Input: part model. Units: mm. Frame: model coordinates. A direction names the side the tool comes from. Round coordinates to 2 decimals unless told otherwise and drop trailing zeros. Write each loop counter-clockwise with the first axis right and the second up, starting at its lowest first coordinate (ties: lowest second). Pieces come first, ordered by that corner, then holes. Notation, with made-up numbers: (-30, 66) -> (-1, 66) arc R17 cw to (-1, 80) -> close; hole circle Ø2 at (-33, -21.5). An arc over 180 degrees is marked (long way). Write item = value, one per line.
Autodesk Inventor part; units mm, degrees
ref_plane "YZ Plane" through (0, 0, 0) normal (1, 0, 0) x (0, 1, 0)
ref_plane "XZ Plane" through (0, 0, 0) normal (0, 1, 0) x (-1, 0, 0)
ref_plane "XY Plane" through (0, 0, 0) normal (0, 0, 1) x (1, 0, 0)
sketch "Sketch1" plane through (0, 0, 0) normal (0, 0, 1) x (1, 0, 0)
  circle A0 centre (29.1378, 0) radius 3.5
  arc A1 (-30.8622, 6) -> (-30.8622, -6) centre (-30.8622, 0) ccw
  arc A2 (29.1378, -6) -> (29.1378, 6) centre (29.1378, 0) ccw
  arc A3 (-30.8622, -6) -> (-27.3004, -4.8284) centre (-30.8622, 0) ccw
  line L0 (-30.8622, 0) -> (-26.6195, -4.2426) construction
  line L1 (-30.8622, 0) -> (-30.8622, -6) construction
  arc A4 (-27.3004, 4.8284) -> (-30.8622, 6) centre (-30.8622, 0) ccw
  line L2 (-30.8622, 0) -> (-26.6195, 4.2426) construction
  line L3 (-30.8622, 0) -> (-30.8622, 6) construction
  arc A5 (29.1378, 6) -> (25.576, 4.8284) centre (29.1378, 0) ccw
  line L4 (29.1378, 0) -> (24.8952, 4.2426) construction
  line L5 (29.1378, 0) -> (29.1378, 6) construction
  arc A6 (25.576, -4.8284) -> (29.1378, -6) centre (29.1378, 0) ccw
  line L6 (29.1378, 0) -> (24.8952, -4.2426) construction
  line L7 (29.1378, 0) -> (29.1378, -6) construction
  line L8 (-25.5195, 4.2426) -> (23.7951, 4.2426)
  line L9 (-25.5195, -4.2426) -> (23.7951, -4.2426)
  arc A7 (-27.3004, 4.8284) -> (-25.5195, 4.2426) centre (-25.5195, 7.2426) ccw
  arc A8 (-25.5195, -4.2426) -> (-27.3004, -4.8284) centre (-25.5195, -7.2426) ccw
  arc A9 (23.7951, 4.2426) -> (25.576, 4.8284) centre (23.7951, 7.2426) ccw
  arc A10 (25.576, -4.8284) -> (23.7951, -4.2426) centre (23.7951, -7.2426) ccw
  line L10 (33.1793, 0) -> (31.1585, -3.5)
  line L11 (31.1585, -3.5) -> (27.1171, -3.5)
  line L12 (27.1171, -3.5) -> (25.0964, 0)
  line L13 (25.0964, 0) -> (27.1171, 3.5)
  line L14 (27.1171, 3.5) -> (31.1585, 3.5)
  line L15 (31.1585, 3.5) -> (33.1793, 0)
  circle A11 centre (-30.8622, 0) radius 1
  point P0 (0, 0)
  point P1 (24.8952, 4.2426)
  dimension "d1" = 7
  dimension "d2" = 60
  dimension "d3" = 6
  dimension "d4" = 6
  dimension "d5" = 45
  dimension "d6" = 45
  dimension "d7" = 45
  dimension "d8" = 45
  dimension "d9" = 3
  dimension "d17" = 2
extrude "Extrusion2" add sketch "Sketch1" along normal blind 3
properties part number "2P.03.01.18.ZW.AileronCrank"
1) Line query: L1, parallel to X at y = 0.75, z = 1.15; L2, parallel to Y at x = -21.5, z = 2.2; L3, parallel to X at y = -2, z = 2.1. Output: solid intervals per line, ascending. Write a range as from..to.
Solutions:
L1 = -36.82..-31.52, -30.2..25.53, 32.75..35.09
L2 = -4.24..4.24
L3 = -36.52..26.25, 32.02..34.79
2) Draft query along Y for faces 6 (the face through (-1, 4.243, 1)), 7 (the face through (-1, 0, 3)), 8 (the face through (29, -3.5, 1)). Return one class per face: +Y half, -Y half, draft (parallel to the pull), parting line (faces both ways), or undercut.
Solutions:
face_6 = +Y half
face_7 = draft
face_8 = undercut
3) Cut plane B-B (y = -2.5). Return the cut outline in (x, z), and give its area (3 significant figures).
Solutions:
outline = (-36.32, 0) -> (26.54, 0) -> (26.54, 3) -> (-36.32, 3) -> close; (31.74, 0) -> (34.59, 0) -> (34.59, 3) -> (31.74, 3) -> close
area = 197 mm^2
4) Cut plane D-D (x = 8). Return the cut outline in (y, z).
Solutions:
outline = (-4.24, 0) -> (4.24, 0) -> (4.24, 3) -> (-4.24, 3) -> close
5) Access query for faces 1 (the face through (-26.444, 4.389, 1.479)), 2 (the face through (29, 3.5, 1)), 3 (the face through (-36.86, -0.13, 1.48)), 4 (the face through (-1, 0, 0)), 5 (the face through (24.72, -4.39, 1.48)). Directions: +Z, -Z, +X, -X, +Y, -Y. A direction counts if a zero-diameter tool reaches every point of the face in a straight line with its end or side. Return the directions, or none.
Solutions:
face_1 = +Z, -Z, +Y
face_2 = +Z, -Z
face_3 = +Z, -Z, -X
face_4 = -Z, +X, -X, +Y, -Y
face_5 = +Z, -Z, -Y
6) Cut plane C-C (x = 30.5). Return the cut outline in (y, z).
Solutions:
outline = (-5.84, 0) -> (-3.5, 0) -> (-3.5, 3) -> (-5.84, 3) -> close; (3.5, 0) -> (5.84, 0) -> (5.84, 3) -> (3.5, 3) -> close
7) Cut plane A-A (z = 1.55). Return the cut outline in (x, y).
Solutions:
outline = (-30.86, -6) arc R6 ccw to (-27.3, -4.83) arc R3 cw to (-25.52, -4.24) -> (23.8, -4.24) arc R3 cw to (25.58, -4.83) arc R6 ccw to (29.14, -6) arc R6 ccw to (29.14, 6) arc R6 ccw to (25.58, 4.83) arc R3 cw to (23.8, 4.24) -> (-25.52, 4.24) arc R3 cw to (-27.3, 4.83) arc R6 ccw to (-30.86, 6) arc R6 ccw to start; hole circle Ø2 at (-30.86, 0); hole (25.1, 0) -> (27.12, -3.5) -> (31.16, -3.5) -> (33.18, 0) -> (31.16, 3.5) -> (27.12, 3.5) -> close
8) First-contact query: P1, Ø1, axis at x = -28, z = 2, coming from the +Y side; P2, Ø1, axis at y = 2.5, z = 2, coming from the +X side; P3, Ø1.5, axis at x = -7.5, z = 2, coming from the +Y side. Flat tips, straight axial feed; report the tip coordinate or a pass-through.
Solutions:
P1 = 5.52
P2 = 34.79
P3 = 4.24
